```python
from build123d import *

# Parameters (mm, degrees)
BOSS_EXTRUDE1_DEPTH = 110
FILLET1_R           = 12
SKETCH2_R           = 6
CUT_EXTRUDE1_DEPTH  = 12
SKETCH3_R           = 6
CUT_EXTRUDE3_DEPTH  = 12
SKETCH4_W           = 60
SKETCH4_H           = 7
CUT_EXTRUDE4_DEPTH  = 60
BOSS_EXTRUDE2_DEPTH = 35
CUT_EXTRUDE5_DEPTH  = 35


with BuildPart() as part:
    # Sketch1 → Boss-Extrude1 (new body)
    with BuildSketch(Plane(origin=(0, 0, 0), x_dir=(0, 0, -1), z_dir=(1, 0, 0))):
        Polygon((10.424266139, 39.165457063), (22.424266139, 39.165457063), (22.424266139, -22.834542937), (-22.575733861, -22.834542937), (-22.575733861, -10.834542937), (10.424266139, -10.834542937), align=None)
    extrude(amount=BOSS_EXTRUDE1_DEPTH)

    # Fillet1
    fillet1_edges = [part.edges().sort_by_distance(p)[0] for p in [
        (110, -16.834542937, 22.575733861),
        (0, -16.834542937, 22.575733861),
        (110, 39.165457063, -16.424266139),
        (0, 39.165457063, -16.424266139),
    ]]
    fillet(fillet1_edges, radius=FILLET1_R)

    # Sketch2 → Cut-Extrude1 (cut)
    with BuildSketch(Plane(origin=(0, -10.834542937, 0), x_dir=(1, 0, 0), z_dir=(0, 1, 0))):
        with Locations(Location((12, -10.575733861, 0), (0, 0, 270))):
            Circle(SKETCH2_R)
        with Locations(Location((98, -10.575733861, 0), (0, 0, 270))):
            Circle(SKETCH2_R)
    extrude(amount=-CUT_EXTRUDE1_DEPTH, mode=Mode.SUBTRACT)

    # Sketch3 → Cut-Extrude3 (cut)
    with BuildSketch(Plane.XY.offset(-10.424266139)):
        with Locations((12, 27.165457063)):
            Circle(SKETCH3_R)
        with Locations((98, 27.165457063)):
            Circle(SKETCH3_R)
    extrude(amount=-CUT_EXTRUDE3_DEPTH, mode=Mode.SUBTRACT)

    # Sketch4 → Cut-Extrude4 (cut)
    with BuildSketch(Plane.XY.offset(22.575733861)):
        with Locations((55, -19.334542937)):
            Rectangle(SKETCH4_W, SKETCH4_H)
    extrude(amount=-CUT_EXTRUDE4_DEPTH, mode=Mode.SUBTRACT)

    # 3DSketch1 → Boss-Extrude2 (add)
    with BuildSketch(Plane(origin=(30, 39.165457063, -22.424266139), x_dir=(0.5843189672224485, -0.8115240874700463, 0), z_dir=(0, 0, 1))):
        with BuildLine():
            Line((0, 0), (5.843189672, 8.115240875))
            ThreePointArc((5.843189672, 8.115240875), (26.780835493, 11.523317678), (23.372758689, 32.460963499))
            Line((23.372758689, 32.460963499), (29.215948361, 40.576204374))
            Line((29.215948361, 40.576204374), (37.331189236, 34.733014701))
            Line((37.331189236, 34.733014701), (34.4095944, 30.675394264))
            Line((34.4095944, 30.675394264), (61.610185565, 0))
            Line((61.610185565, 0), (48.755168287, -17.853529924))
            Line((48.755168287, -17.853529924), (11.036835711, -1.785569235))
            Line((11.036835711, -1.785569235), (8.115240875, -5.843189672))
            Line((8.115240875, -5.843189672), (0, 0))
        make_face()
    extrude(amount=BOSS_EXTRUDE2_DEPTH)

    # Sketch5 → Cut-Extrude5 (cut)
    with BuildSketch(Plane.XY.offset(-10.424266139)):
        with BuildLine():
            Line((40, 39.165457063), (70, 39.165457063))
            ThreePointArc((70, 39.165457063), (55, 24.165457063), (40, 39.165457063))
        make_face()
    extrude(amount=-CUT_EXTRUDE5_DEPTH, mode=Mode.SUBTRACT)


solid = part.part
```
The listing builds one solid part. Answer for the finished solid, in the listing's coordinates (mm). A direction names the side the tool comes from. Round coordinates to 2 decimals unless told otherwise and drop trailing zeros. Loops run counter-clockwise (first coordinate to the right, second up) from the corner with the lowest first, then second, coordinate; pieces in that order, holes last.
Q1. Section C-C, the plane y = 16.5 is taken. Determine the outline of the cut face in (x, z), then the cut area to 3 significant figures.
Q2. Find the intervals of material crossed by line 1 (Z direction, x = 36.5, y = 7); line 2 (Y direction, x = 98, z = -15); line 3 (X direction, y = -18.5, z = -6.5), in increasing order.
Q3. Section A-A, the plane z = -2.5 is taken. Determine the outline of the cut face in (x, y), then the cut area to 3 significant figures.
Q4. Which of the six approach directions +Z, -Z, +X, -X, +Y, -Y give full straight-line access (tool end or side, diameter ignored) to faces 4 (the face through (70.563, 9.446, 0.915)), 5 (the face through (80, 34, 1)), 6 (the face through (30, 34, 1))?
Q5. For a pull along Y with two mould halves and no side action, classify faces 1 (the face through (103.95, -16.75, 9.79)), 2 (the face through (39.563, 8.886, 0.915)), 3 (the face through (3.609, 35.744, -16.508)) as released by +Y, released by -Y, zero draft, split by the parting line, or undercut.
Q6. Given pin 1 Ø15 at (x, y) = (53, 11) entering from +Z; pin 2 Ø2.5 at (x, z) = (78, -0.5) entering from -Y; pin 3 Ø6 at (y, z) = (26, -1.5) entering from +X; pin 4 Ø14 at (x, y) = (12, 27.17) entering from -Z, each flat-ended and moving along its own axis, determine where each tip first touches the part or whether it passes through.
Completed:
1. outline: (0, -22.42) - (110, -22.42) - (110, -10.42) - (72.15, -10.42) - (72.15, 12.58) - (37.85, 12.58) - (37.85, -10.42) - (0, -10.42) - close
1. area: 2,110 mm2
2. line 1: z = -22.42 to -10.42
2. line 2: y = -22.83 to 21.17, 33.17 to 39.17
2. line 3: x = 0 to 25, 85 to 110
3. outline: (0, -22.83) - (25, -22.83) - (25, -15.83) - (85, -15.83) - (85, -22.83) - (110, -22.83) - (110, -10.83) - (0, -10.83) - close; (30, 29.17) - (35, 29.17) - (44, -10.83) - (66, -10.83) - (75, 29.17) - (80, 29.17) - (80, 39.17) - (70, 39.17) arc R15 cw to (40, 39.17) - (30, 39.17) - close
3. area: 2,290 mm2
4. face 4: +Z, +X
4. face 5: +Z, +X, +Y
4. face 6: +Z, -X, +Y
5. face 1: zero draft
5. face 2: undercut
5. face 3: released by +Y
6. pin 1: stops at z = 12.58
6. pin 2: stops at y = -15.83
6. pin 3: stops at x = 74.96
6. pin 4: stops at z = -22.42
